from build123d import *

# Parameters (mm, degrees)
SKETCH_1_W          = 25
SKETCH_1_H          = 25
SKETCH_1_W_2        = 15
SKETCH_1_H_2        = 15
EXTRUDE_1_DEPTH     = 30
SKETCH_2_W          = 25
SKETCH_2_H          = 18
SKETCH_2_W_2        = 10
SKETCH_2_H_2        = 3
EXTRUDE_2_DEPTH     = 30
SKETCH_3_R          = 1.65
CUT_EXTRUDE_1_DEPTH = 30
SKETCH_4_R          = 1.65
CUT_EXTRUDE_2_DEPTH = 1000
FILLET_1_R          = 1


with BuildPart() as part:
    # 草图1 → 凸台-拉伸1 (new body)
    with BuildSketch(Plane.XY):
        Rectangle(SKETCH_1_W, SKETCH_1_H)
        Rectangle(SKETCH_1_W_2, SKETCH_1_H_2, mode=Mode.SUBTRACT)
    extrude(amount=EXTRUDE_1_DEPTH)

    # 草图2 → 凸台-拉伸2 (add)
    with BuildSketch(Plane.XY.offset(30)):
        with Locations((0, -21.5)):
            Rectangle(SKETCH_2_W, SKETCH_2_H)
        with Locations((-17.5, -32)):
            Rectangle(SKETCH_2_W_2, SKETCH_2_H_2)
        with Locations((0, -32)):
            Rectangle(SKETCH_2_W, SKETCH_2_H_2)
        with Locations((17.5, -32)):
            Rectangle(SKETCH_2_W_2, SKETCH_2_H_2)
    extrude(amount=-EXTRUDE_2_DEPTH)

    # 草图3 → 切除-拉伸1 (cut)
    with BuildSketch(Plane(origin=(0, -30.5, 0), x_dir=(1, 0, 0), z_dir=(0, 1, 0))):
        with Locations(Location((17.5, -15, 0), (0, 0, 270))):
            Circle(SKETCH_3_R)
    cut_extrude_1 = extrude(amount=-CUT_EXTRUDE_1_DEPTH, mode=Mode.SUBTRACT)

    # 镜向1: 切除-拉伸1 across plane
    add(cut_extrude_1.mirror(Plane(origin=(0, 0, 0), x_dir=(0, 0, 1), z_dir=(1, 0, 0))), mode=Mode.SUBTRACT)

    # 草图4 → 切除-拉伸2 (cut)
    with BuildSketch(Plane(origin=(0, 12.5, 0), x_dir=(1, 0, 0), z_dir=(0, 1, 0))):
        with Locations(Location((0, -15, 0), (0, 0, 270))):
            Circle(SKETCH_4_R)
    extrude(amount=-CUT_EXTRUDE_2_DEPTH, mode=Mode.SUBTRACT)

    # 圆角1
    fillet_1_edges = [part.edges().sort_by_distance(p)[0] for p in [
        (-12.5, -30.5, 15),
        (12.5, -30.5, 15),
        (-12.5, 12.5, 15),
        (12.5, 12.5, 15),
    ]]
    fillet(fillet_1_edges, radius=FILLET_1_R)


solid = part.part
Verification items for the finished model (mm, model axes). A direction names the side the tool comes from. Give positions to 0.01 mm unless a question says otherwise; leave off trailing zeros. Write each loop counter-clockwise with the first axis right and the second up, starting at its lowest first coordinate (ties: lowest second). Pieces come first, ordered by that corner, then holes. Notation, with made-up numbers: M 27,-39 L 64,-39 A33 ccw 64,-5 Z; hole C -38.5,-14.5 d7. An arc over 180 degrees is marked long. Use CSV: the item, a comma, the result in double quotes.
1) Cross-section at B-B (y = -0.5). Enter the section's corners in (x, z).
Final values:
outline,"M -12.5,0 L -7.5,0 L -7.5,30 L -12.5,30 Z; M 7.5,0 L 12.5,0 L 12.5,30 L 7.5,30 Z"
2) Go/stop test with flat-tipped pins: pin 1 Ø9 at (y, z) = (-6, 21.5) entering from +X; pin 2 Ø10 at (y, z) = (-18.5, 15) entering from -X; pin 3 Ø4 at (x, z) = (-17.5, 15) entering from +Y. Record where each tip stops, or that it passes through.
Final values:
pin 1,"x = 12.5"
pin 2,"x = -12.5"
pin 3,"y = -30.5"
3) Cross-section at A-A (z = 15). State how many separate pieces and enclosed holes the cut face has, plus the area to 3 significant figures.
Final values:
separate pieces,"4"
enclosed holes,"0"
area,"863 mm²"
4) Material ranges on line 1 along X through (y, z) = (-32.25, 15); line 2 along Z through (x, y) = (-17.5, -31.5); line 3 along Y through (x, z) = (4, 8.5), recorded low to high.
Final values:
line 1,"-22.5 to -19.15, -15.85 to -1.65, 1.65 to 15.85, 19.15 to 22.5"
line 2,"0 to 13.35, 16.65 to 30"
line 3,"-33.5 to -7.5, 7.5 to 12.5"
5) Release check for a two-part mould opening along X. For faces 1 (the face through (-22.5, -32, 15)), 2 (the face through (0.496, 10.035, 16.574)), 3 (the face through (-2, -7.5, 15)), 4 (the face through (0, -33.5, 19)) record: released by +X, released by -X, zero draft, split by the parting line, or undercut.
Final values:
face 1,"released by -X"
face 2,"undercut"
face 3,"undercut"
face 4,"zero draft"
6) Cross-section at C-C (x = 0). Enter the section's corners in (y, z).
Final values:
outline,"M -33.5,0 L -7.5,0 L -7.5,13.35 L -33.5,13.35 Z; M -33.5,16.65 L -7.5,16.65 L -7.5,30 L -33.5,30 Z; M 7.5,0 L 12.5,0 L 12.5,13.35 L 7.5,13.35 Z; M 7.5,16.65 L 12.5,16.65 L 12.5,30 L 7.5,30 Z"
7) Access from +Z, -Z, +X, -X, +Y, -Y to the whole of each face (thin tool, end or side, straight path). Record for faces 5 (the face through (-12.5, -9, 15)), 6 (the face through (-2, 7.5, 15)), 7 (the face through (12.5, -9, 15)).
Final values:
face 5,"+Z, -Z, -X, +Y"
face 6,"+Z, -Z"
face 7,"+Z, -Z, +X, +Y"
8) Cross-section at D-D (x = 5). Enter the section's corners in (y, z), plus the area to 3 significant figures.
Final values:
outline,"M -33.5,0 L -7.5,0 L -7.5,30 L -33.5,30 Z; M 7.5,0 L 12.5,0 L 12.5,30 L 7.5,30 Z"
area,"930 mm²"
